Geometry: final body of the model. Coordinates: model frame, mm. A direction names the side the tool comes from. Give positions to 0.01 mm unless a question says otherwise; leave off trailing zeros. Write each loop counter-clockwise with the first axis right and the second up, starting at its lowest first coordinate (ties: lowest second). Pieces come first, ordered by that corner, then holes. Notation, with made-up numbers: M 75.25,29.5 L 101.25,29.5 A33 ccw 101.25,58.5 Z; hole C -4.5,9.25 d6. An arc over 180 degrees is marked long. Use a Markdown table: item, result. Add a question column.
1) Line query: line 1 (X direction, y = 3, z = 0); line 2 (Y direction, x = -51.5, z = -56.5); line 3 (Z direction, x = 18, y = 2). Output: solid intervals per line, ascending.
2) Section D-D on z = 59.5. Return the cut outline in (x, y).
3) Pin query (flat end, axial travel): pin 1 (1.5 mm diameter, centred on x = 9.5, z = -22.5, fed in from -Y). Return the tip coordinate at first contact, or that it passes through.
4) Section C-C on y = 1.5. Return the cut outline in (x, z), then the cut area to 3 significant figures.
5) Section B-B on x = 0. Return the cut outline in (y, z), then the cut area to 3 significant figures.
6) Section A-A on z = 0. Return the cut outline in (x, y), then the cut area to 3 significant figures.
7) Draft query along X for faces 3 (the flat face through (67.5, 2, 1)), 4 (the flat face through (-67.5, 2, 1)), 5 (the cylindrical face through (13.67, -2.22, 63.22)), 6 (the flat face through (53, -4.5, 59)). Return one class per face: +X half, -X half, draft (parallel to the pull), parting line (faces both ways), or undercut.
8) Set-up query: faces 1 (the cylindrical face through (56.367, -2.218, 58.992)), 2 (the flat face through (13, -4.5, 59)). Return all of +Z, -Z, +X, -X, +Y, -Y with unobstructed straight access to the full face (end or side cutting, diameter ignored); none if empty.
```python
from build123d import *

# Parameters (mm, degrees)
SKETCH1_W           = 135
SKETCH1_H           = 135
SKETCH1_R           = 3.9
BOSS_EXTRUDE1_DEPTH = 4
SKETCH1_3_R         = 3.9
BOSS_EXTRUDE2_DEPTH = 4.5
SKETCH2_R           = 25
CUT_EXTRUDE1_DEPTH  = 10


with BuildPart() as part:
    # Sketch1 → Boss-Extrude1 (new body)
    # profile 1 of 3: a face of its own
    with BuildSketch(Plane(origin=(0, 0, 0), x_dir=(1, 0, 0), z_dir=(0, 1, 0))):
        Rectangle(SKETCH1_W, SKETCH1_H)
        with Locations((52.5, -59.5)):
            Circle(SKETCH1_R, mode=Mode.SUBTRACT)
        with Locations((12.5, -59.5)):
            Circle(SKETCH1_R, mode=Mode.SUBTRACT)
    # profile 2 of 3: a face of its own
    with BuildSketch(Plane(origin=(0, 0, 0), x_dir=(1, 0, 0), z_dir=(0, 1, 0))):
        with Locations((52.5, -59.5)):
            Circle(SKETCH1_R)
    # profile 3 of 3: a face of its own
    with BuildSketch(Plane(origin=(0, 0, 0), x_dir=(1, 0, 0), z_dir=(0, 1, 0))):
        with Locations((12.5, -59.5)):
            Circle(SKETCH1_R)
    extrude(amount=BOSS_EXTRUDE1_DEPTH)

    # Sketch1_3 → Boss-Extrude2 (add)
    with BuildSketch(Plane(origin=(0, 0, 0), x_dir=(1, 0, 0), z_dir=(0, 1, 0))):
        with Locations(Location((12.5, -59.5, 0), (0, 0, 270))):
            Circle(SKETCH1_3_R)
        with Locations(Location((52.5, -59.5, 0), (0, 0, 270))):
            Circle(SKETCH1_3_R)
    extrude(amount=-BOSS_EXTRUDE2_DEPTH)

    # Sketch2 → Cut-Extrude1 (cut)
    with BuildSketch(Plane(origin=(0, 4, 0), x_dir=(1, 0, 0), z_dir=(0, 1, 0))):
        with Locations(Location((0, 0, 0), (0, 0, 270))):
            Circle(SKETCH2_R)
    extrude(amount=-CUT_EXTRUDE1_DEPTH, mode=Mode.SUBTRACT)


solid = part.part
```
Found:
| question | item | result |
|---|---|---|
| 1 | line 1 | -67.5 to -25, 25 to 67.5 |
| 1 | line 2 | 0 to 4 |
| 1 | line 3 | -67.5 to -17.35, 17.35 to 67.5 |
| 2 | outline | M -67.5,0 L 8.6,0 L 8.6,-4.5 L 16.4,-4.5 L 16.4,0 L 48.6,0 L 48.6,-4.5 L 56.4,-4.5 L 56.4,0 L 67.5,0 L 67.5,4 L -67.5,4 Z |
| 3 | pin 1 | y = 0 |
| 4 | outline | M -67.5,-67.5 L 67.5,-67.5 L 67.5,67.5 L -67.5,67.5 Z; hole C 0,0 d50 |
| 4 | area | 16,300 mm² |
| 5 | outline | M 0,-67.5 L 4,-67.5 L 4,-25 L 0,-25 Z; M 0,25 L 4,25 L 4,67.5 L 0,67.5 Z |
| 5 | area | 340 mm² |
| 6 | outline | M -67.5,0 L -25,0 L -25,4 L -67.5,4 Z; M 25,0 L 67.5,0 L 67.5,4 L 25,4 Z |
| 6 | area | 340 mm² |
| 7 | face 3 | +X half |
| 7 | face 4 | -X half |
| 7 | face 5 | undercut |
| 7 | face 6 | draft |
| 8 | face 1 | -Y |
| 8 | face 2 | +Z, -Z, +X, -X, -Y |
